Geometry check sheet. Reference: the model listing, model coordinates, mm. Face numbers are marked on the shaded views. Round coordinates to 2 decimals unless told otherwise and drop trailing zeros. Order: outer loops, then holes, each group sorted by start corner. A loop starts at its lowest first (then second) coordinate and runs counter-clockwise, first axis right, second up. Notation, with made-up numbers: (69, 19) - (101, 19) arc R29 ccw to (101, 57) - close; hole circle Ø4 at (-23, -26). An arc over 180 degrees is marked (long way). One line per question, with ' | ' between items. Start each with the question number.
Q1. Sectioned sample at B-B, the plane x = 0. Enter the section's corners in (y, z), then the cut area to 3 significant figures.
Q2. Sectioned sample at C-C, the plane y = 58. Enter the section's corners in (x, z).
Q3. Sectioned sample at A-A, the plane z = 0. Enter the section's corners in (x, y).
Q4. Gauge pin test, flat ends, axial feed: P1, Ø6, axis at y = 96.5, z = -21.5, coming from the +X side; P2, Ø2, axis at y = 14.5, z = 30.5, coming from the -X side; P3, Ø2, axis at x = 10.5, y = 67, coming from the +Z side. Record the tip position at first contact, or that the pin passes through.
Q5. Mould release check, pull along X, two halves, no side actions. Record for the marked faces 1, 2 and 3: +X half, -X half, draft (parallel to the pull), parting line (faces both ways), or undercut.
Q6. Material ranges on line 1 along X through (y, z) = (21, -1); line 2 along Y through (x, z) = (-6, -30.5); line 3 along Z through (x, y) = (-14, 65), recorded low to high.
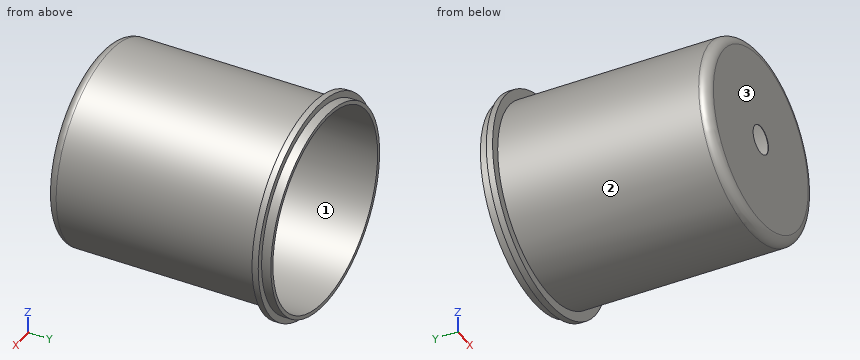
Autodesk Inventor part; units mm, degrees
ref_plane "YZ Plane" through (0, 0, 0) normal (1, 0, 0) x (0, 1, 0)
ref_plane "XZ Plane" through (0, 0, 0) normal (0, 1, 0) x (-1, 0, 0)
ref_plane "XY Plane" through (0, 0, 0) normal (0, 0, 1) x (1, 0, 0)
sketch "Sketch1" plane through (0, 0, 0) normal (0, 0, 1) x (1, 0, 0)
  line L0 (46.8, 0) -> (47, 0)
  line L1 (47, 4.6) -> (47, 101.7)
  line L2 (47, 109.2) -> (46.8, 109.2)
  line L3 (46.8, 109.2) -> (46.8, 4.8)
  line L4 (46.8, 109.2) -> (48.6, 109.2)
  line L5 (48.6, 109.2) -> (48.6, 104.7)
  line L6 (48.6, 104.7) -> (51.6, 104.7)
  line L7 (51.6, 104.7) -> (51.6, 101.7)
  line L8 (51.6, 101.7) -> (48.6, 101.7)
  line L9 (48.6, 101.7) -> (47, 101.7)
  line L10 (0, 0) -> (0, 20.8136)
  line L11 (42.4, 0) -> (-0.2292, 0)
  line L12 (0, 0) -> (0, 0.2)
  line L13 (0, 0.2) -> (42.2, 0.2)
  arc A0 (42.2, 0.2) -> (46.8, 4.8) centre (42.2, 4.8) ccw
  arc A1 (42.4, 0) -> (47, 4.6) centre (42.4, 4.6) ccw
  dimension "d1" = 0.2
  dimension "d2" = 109.2
  dimension "d3" = 1.8
  dimension "d4" = 4.5
  dimension "d5" = 3
  dimension "d6" = 3
  dimension "d7" = 0.2
  dimension "d8" = 90
  dimension "d9" = 4.6
revolve "Revolution1" add sketch "Sketch1" angle 360 about axis through (0, 0, 0) along (0, 1, 0)
sketch "Sketch2" plane through (0, 0, 0) normal (0, -1, 0) x (1, 0, 0)
  circle A0 centre (0, 0) radius 6.858
  dimension "d11" = 13.716
extrude "Extrusion1" cut sketch "Sketch2" against normal blind 1
properties part number "ContenedorTest"
Determined:
1) outline: (0, -42.4) arc R4.6 ccw to (4.6, -47) - (101.7, -47) - (101.7, -51.6) - (104.7, -51.6) - (104.7, -48.6) - (109.2, -48.6) - (109.2, -46.8) - (4.8, -46.8) arc R4.6 cw to (0.2, -42.2) - (0.2, -6.86) - (0, -6.86) - close; (0, 6.86) - (0.2, 6.86) - (0.2, 42.2) arc R4.6 cw to (4.8, 46.8) - (109.2, 46.8) - (109.2, 48.6) - (104.7, 48.6) - (104.7, 51.6) - (101.7, 51.6) - (101.7, 47) - (4.6, 47) arc R4.6 ccw to (0, 42.4) - close | area: 102 mm2
2) outline: circle Ø94 at (0, 0); hole circle Ø93.6 at (0, 0)
3) outline: (-51.6, 101.7) - (-47, 101.7) - (-47, 4.6) arc R4.6 ccw to (-42.4, 0) - (-6.86, 0) - (-6.86, 0.2) - (-42.2, 0.2) arc R4.6 cw to (-46.8, 4.8) - (-46.8, 109.2) - (-48.6, 109.2) - (-48.6, 104.7) - (-51.6, 104.7) - close; (6.86, 0) - (42.4, 0) arc R4.6 ccw to (47, 4.6) - (47, 101.7) - (51.6, 101.7) - (51.6, 104.7) - (48.6, 104.7) - (48.6, 109.2) - (46.8, 109.2) - (46.8, 4.8) arc R4.6 cw to (42.2, 0.2) - (6.86, 0.2) - close
4) P1: stops at x = 43.21 | P2: stops at x = -36.59 | P3: stops at z = 46.03
5) face 1: undercut | face 2: parting line | face 3: draft
6) line 1: x = -46.99 to -46.79, 46.79 to 46.99 | line 2: y = 0 to 0.2 | line 3: z = -44.87 to -44.66, 44.66 to 44.87
